Here's how the part is built. I have some questions about the finished solid (model axes, mm). A direction names the side the tool comes from. Round coordinates to 2 decimals unless told otherwise and drop trailing zeros. Write each loop counter-clockwise with the first axis right and the second up, starting at its lowest first coordinate (ties: lowest second). Pieces come first, ordered by that corner, then holes. Notation, with made-up numbers: (-30.5, 28.5) - (27.5, 28.5) arc R18 cw to (27.5, 61.5) - close; hole circle Ø2 at (4.5, -0.75). An arc over 180 degrees is marked (long way). One line per item, written item: value. Start each with the question number.
Item 1: Imagine slicing it at A-A, the plane y = 7.25. Please give me the cut outline in (x, z).
Item 2: Imagine slicing it at B-B, the plane x = 0. Please give me the cut outline in (y, z), then the cut area to 3 significant figures.
Item 3: For P1, Ø1.8, axis at y = 9.5, z = -3.5, coming from the -X side; P2, Ø0.8, axis at x = 0, y = 6.5, coming from the -Z side; P3, Ø4, axis at y = 8.5, z = -4.5, coming from the +X side, each with a flat end and sliding along its axis, tell me the tip position at first contact or that it passes through.
Item 4: For faces 4 (the face through (-0.03, 14.2, 1.25)), 5 (the face through (0, 12, 0)), 6 (the face through (-0.1, 0, -3.4)), 7 (the face through (0, 9, -6.604)), which set-ups out of +Z, -Z, +X, -X, +Y, -Y let a thin tool reach every point of the face, with its end or its side?
Item 5: Imagine slicing it at C-C, the plane y = 3. Please give me the cut outline in (x, z).
Item 6: If I drill on line 1 (X direction, y = 8.5, z = 0); line 2 (Y direction, x = 3, z = -4.25); line 3 (X direction, y = 6.25, z = 0), over which ranges is the centre line in solid material (lowest first)?
Item 7: Thinking about a two-plate mould opening in X: for faces 1 (the face through (-0.25, 8.93, 5.98)), 2 (the face through (1, 13.9, 1)), 3 (the face through (0.9, 5.92, 2.86)), which applies, released by +X, released by -X, zero draft, split by the parting line, or undercut?
```python
from build123d import *

# Parameters (mm, degrees)
BOSS_EXTRUDE1_REACH             = 19.922
BOSS_EXTRUDE1_DIRECTION_2_DEPTH = 0.6
SKETCH3_R                       = 3
CUT_EXTRUDE1_DEPTH              = 12


with BuildPart() as part:
    # Sketch1 → Revolve1 (revolve)
    with BuildSketch(Plane.XY, mode=Mode.PRIVATE) as revolve1_sk:
        Polygon((0, 13.9), (5.55, 13.9), (6.408097327, 4.091902673), (8, 2.5), (8, 0), (0, 0), align=None)
    revolve(revolve1_sk.sketch.rotate(Axis((0, 0, 0), (0, 1, 0)), 90), axis=Axis((0, 0, 0), (0, 1, 0)))

    # Sketch2 → Boss-Extrude1 (add, up to next)
    with BuildSketch(Plane(origin=(0, 13.9, 0), x_dir=(1, 0, 0), z_dir=(0, 1, 0)), mode=Mode.PRIVATE) as boss_extrude1_sk1:
        with BuildLine():
            Line((-1.25000004, 6.104), (-1.25000004, 0))
            ThreePointArc((-1.25000004, 0), (0, -1.25000004), (1.25000004, 0))
            Line((1.25000004, 0), (1.25000004, 6.104))
            ThreePointArc((1.25000004, 6.104), (1.103553431, 6.457553391), (0.75000004, 6.604))
            Line((0.75000004, 6.604), (-0.75000004, 6.604))
            ThreePointArc((-0.75000004, 6.604), (-1.103553431, 6.457553391), (-1.25000004, 6.104))
        make_face()
    boss_extrude1_tool1 = extrude(boss_extrude1_sk1.sketch, amount=-BOSS_EXTRUDE1_REACH, mode=Mode.PRIVATE) - part.part
    add(boss_extrude1_tool1.solids().sort_by_distance((0, 13.9, -2.78502))[0])

    # Sketch2 → Boss-Extrude1 direction 2 (add)
    with BuildSketch(Plane(origin=(0, 13.9, 0), x_dir=(1, 0, 0), z_dir=(0, 1, 0))):
        with BuildLine():
            Line((-1.25000004, 6.104), (-1.25000004, 0))
            ThreePointArc((-1.25000004, 0), (0, -1.25000004), (1.25000004, 0))
            Line((1.25000004, 0), (1.25000004, 6.104))
            ThreePointArc((1.25000004, 6.104), (1.103553431, 6.457553391), (0.75000004, 6.604))
            Line((0.75000004, 6.604), (-0.75000004, 6.604))
            ThreePointArc((-0.75000004, 6.604), (-1.103553431, 6.457553391), (-1.25000004, 6.104))
        make_face()
    extrude(amount=BOSS_EXTRUDE1_DIRECTION_2_DEPTH)

    # Sketch3 → Cut-Extrude1 (cut)
    with BuildSketch(Plane(origin=(0, 0, 0), x_dir=(1, 0, 0), z_dir=(0, 1, 0))):
        with Locations(Location((0, 0, 0), (0, 0, 270))):
            Circle(SKETCH3_R)
    extrude(amount=CUT_EXTRUDE1_DEPTH, mode=Mode.SUBTRACT)


solid = part.part
```
Values follow:
1. outline: (-1.25, -6.1) arc R0.5 ccw to (-0.75, -6.6) - (0.75, -6.6) arc R0.5 ccw to (1.25, -6.1) - (1.25, -6) arc R6.13 ccw (long way) to (-1.25, -6) - close; hole circle Ø6 at (0, 0)
2. outline: (0, -8) - (2.5, -8) - (3.9, -6.6) - (14.5, -6.6) - (14.5, 1.25) - (13.9, 1.25) - (13.9, 5.55) - (4.09, 6.41) - (2.5, 8) - (0, 8) - (0, 3) - (12, 3) - (12, -3) - (0, -3) - close
2. area: 119 mm^2
3. P1: stops at x = -5.34
3. P2: stops at z = -6.6
3. P3: stops at x = 5.5
4. face 4: +Z, +Y
4. face 5: -Y
4. face 6: +Z, -Z, +X, -X, -Y
4. face 7: -Z, +X, -X, +Y
5. outline: circle Ø15 at (0, 0); hole circle Ø6 at (0, 0)
6. line 1: x = -6.02 to -3, 3 to 6.02
6. line 2: y = 0 to 13.9
6. line 3: x = -6.22 to -3, 3 to 6.22
7. face 1: split by the parting line
7. face 2: zero draft
7. face 3: undercut
